from build123d import *

# Parameters (mm, degrees)
F1_DEPTH = 3


with BuildPart() as f1:
    # F0 (on Front) → F1 (new body)
    with BuildSketch(Plane.XZ):
        with BuildLine():
            Line((1.45, 0), (1.45, -34.969951))
            ThreePointArc((1.45, -34.969951), (34.992487, 0.725156), (0, 35))
            ThreePointArc((0, 35), (-34.992487, 0.725156), (-1.45, -34.969951))
            Line((-1.45, -34.969951), (-1.45, 0))
            Line((-1.45, 0), (0, 0))
            Line((0, 0), (1.45, 0))
        make_face()
    extrude(amount=F1_DEPTH)


solid = f1.part
Design review of the part built by this model. Coordinates are the model's own, in mm. A direction names the side the tool comes from. Round coordinates to 2 decimals unless told otherwise and drop trailing zeros. Order: outer loops, then holes, each group sorted by start corner. A loop starts at its lowest first (then second) coordinate and runs counter-clockwise, first axis right, second up. Notation, with made-up numbers: M 75,24.5 L 115,24.5 A36 ccw 115,60.5 Z; hole C 39.5,62 d9. An arc over 180 degrees is marked long. Answer as CSV lines item,"result". Start each with the question number.
1) Add section C-C (x = 21). Give the boundary of the cut face in (y, z).
2) Add section D-D (z = -13). Give the boundary of the cut face in (x, y), then the cut area to 3 significant figures.
3) Add section B-B (y = -1.7). Give the boundary of the cut face in (x, z).
4) Add section A-A (z = -24). Give the boundary of the cut face in (x, y), then the cut area to 3 significant figures.
5) The part is to be moulded in two halves that separate along X. For faces 1 (the face through (0, -1, 0)), 2 (the face through (1.45, -1, -17)), 3 (the face through (0, -3, 1)), say which applies: +X half, -X half, draft (parallel to the pull), parting line (faces both ways), or undercut.
6) For pin 1 Ø1.4 at (x, y) = (0.5, -1) entering from -Z; pin 2 Ø0.9 at (y, z) = (-1.5, -10) entering from -X, all flat-tipped, find the tip position at first contact; note any pin that passes through.
7) Tool access review of faces 4 (the face through (-1.45, -1, -18)), 5 (the face through (0, 0, 1)): name each direction out of +Z, -Z, +X, -X, +Y, -Y from which nothing blocks a thin tool from reaching the whole face with its end or side.
8) Wall thickness on line 1 along X through (y, z) = (-1.15, -6.5); line 2 along X through (y, z) = (-1.25, -6); line 3 along Z through (x, y) = (1, -0.35): over which ranges is each line inside the solid? List them lowest first. Write a range as [from, to].
Resolved:
1,outline,"M -3,-28 L 0,-28 L 0,28 L -3,28 Z"
2,outline,"M -32.5,-3 L -1.45,-3 L -1.45,0 L -32.5,0 Z; M 1.45,-3 L 32.5,-3 L 32.5,0 L 1.45,0 Z"
2,area,"186 mm^2"
3,outline,"M -1.45,-34.97 L -1.45,0 L 1.45,0 L 1.45,-34.97 A35 ccw long Z"
4,outline,"M -25.48,-3 L -1.45,-3 L -1.45,0 L -25.48,0 Z; M 1.45,-3 L 25.48,-3 L 25.48,0 L 1.45,0 Z"
4,area,"144 mm^2"
5,face 1,"undercut"
5,face 2,"undercut"
5,face 3,"draft"
6,pin 1,"z = 0"
6,pin 2,"x = -33.67"
7,face 4,"-Z, +Y, -Y"
7,face 5,"+Z, -Z, +X, -X, +Y"
8,line 1,"[-34.39, -1.45], [1.45, 34.39]"
8,line 2,"[-34.48, -1.45], [1.45, 34.48]"
8,line 3,"[0, 34.99]"
